```python
from build123d import *

# Parameters (mm, degrees)
F0_W     = 220
F0_H     = 220
F1_DEPTH = 3
F2_W     = 40
F2_H     = 160
F2_R     = 2
F3_DEPTH = 25
F4_SIZE  = 19.99999
F5_R     = 2
F6_DEPTH = 25


# Not quite as in the source:
# - a fillet or chamfer is up to 0.001 mm smaller than in the source, because OpenCascade refuses the exact size
# - a pattern or mirror of a feature is missing from the dataset's text; its kind, count and spacing are read off the source's solid


with BuildPart() as f1:
    # F0 (on Top) → F1 (new body)
    with BuildSketch(Plane.XY):
        Rectangle(F0_W, F0_H)
    extrude(amount=F1_DEPTH)

    # F2 (on face) → F3 (cut)
    with BuildSketch(Plane.XY.offset(3)):
        with Locations((-90, 0)):
            Rectangle(F2_W, F2_H)
        with Locations((105, 105)):
            Circle(F2_R)
        with Locations((105, -105)):
            Circle(F2_R)
        with Locations((-105, 105)):
            Circle(F2_R)
        with Locations((-105, -105)):
            Circle(F2_R)
    f3 = extrude(amount=-F3_DEPTH, mode=Mode.SUBTRACT)

    # F3_copies: F3 across plane
    add(f3.mirror(Plane(origin=(0, 0, 0), x_dir=(0, 0, 1), z_dir=(1, 0, 0))), mode=Mode.SUBTRACT)

    # F4 (size 20 in the source; OpenCascade refuses exactly that, so slightly less here)
    f4_edges = [f1.edges().sort_by_distance(p)[0] for p in [
        (-110, 80, 1.5),
        (-110, -80, 1.5),
        (-70, -80, 1.5),
        (-70, 80, 1.5),
        (110, 80, 1.5),
        (70, 80, 1.5),
        (70, -80, 1.5),
        (110, -80, 1.5),
    ]]
    chamfer(f4_edges, length=F4_SIZE)

    # F5 (on face) → F6 (cut)
    with BuildSketch(Plane(origin=(0, 0, 0), x_dir=(1, 0, 0), z_dir=(0, 0, -1))):
        with Locations((-47, 100)):
            Circle(F5_R)
        with Locations((-47, -40)):
            Circle(F5_R)
        with Locations((47, -40)):
            Circle(F5_R)
        with Locations((47, 100)):
            Circle(F5_R)
    extrude(amount=-F6_DEPTH, mode=Mode.SUBTRACT)


solid = f1.part
```
Build history of the part. All positions in model axes, mm. A direction names the side the tool comes from. Give positions to 0.01 mm unless a question says otherwise; leave off trailing zeros. Loops run counter-clockwise (first coordinate to the right, second up) from the corner with the lowest first, then second, coordinate; pieces in that order, holes last.
Item 1: Slice it at C-C, the plane y = 35. List the corners of the cut face in (x, z).
Answers follow:
outline: (-70, 0) - (70, 0) - (70, 3) - (-70, 3) - close
Item 2: Flat gauge pins, fed straight in: pin 1 (2.5 mm diameter, centred on x = -105, y = 105, fed in from +Z); pin 2 (1.5 mm diameter, centred on y = 20, z = 1.5, fed in from -X); pin 3 (0.9 mm diameter, centred on y = -4.5, z = 1.5, fed in from +X); pin 4 (1.5 mm diameter, centred on y = -62.5, z = 1, fed in from +X). Where does each tip first touch, or does it go through?
Answers follow:
pin 1: passes through
pin 2: stops at x = -70
pin 3: stops at x = 70
pin 4: stops at x = 73.25
Item 3: Slice it at B-B, the plane z = 1.8. Give the number of separate pieces and of enclosed holes in the cut face, and give its area (3 significant figures).
Answers follow:
separate pieces: 1
enclosed holes: 8
area: 35,500 mm2
Item 4: Pull direction Y, two halves, no side cores. Call faces 1 (the face through (100, 90, 2)), 2 (the face through (-2, 2, 0)): released by +Y, released by -Y, zero draft, split by the parting line, or undercut.
Answers follow:
face 1: undercut
face 2: zero draft
Item 5: Slice it at A-A, the plane x = -80.5. List the corners of the cut face in (y, z).
Answers follow:
outline: (-110, 0) - (-70.5, 0) - (-70.5, 3) - (-110, 3) - close; (70.5, 0) - (110, 0) - (110, 3) - (70.5, 3) - close
Item 6: Drill centre lines: line 1 (X direction, y = 40, z = 0.8); line 2 (X direction, y = -105, z = 1.1); line 3 (Y direction, x = 47, z = 1.95). Where is each one in solid material? Low to high.
Answers follow:
line 1: x = -70 to -49, -45 to 45, 49 to 70
line 2: x = -110 to -107, -103 to 103, 107 to 110
line 3: y = -110 to -102, -98 to 38, 42 to 110
Item 7: Which spindle directions (+Z, -Z, +X, -X, +Y, -Y) get a long thin tool onto all of the face, cutting with end or side? Do faces 3 (the face through (-2, 2, 3)), 4 (the face through (80, 70, 2)), 5 (the face through (-100, -90, 2)). Say none if no direction does.
Answers follow:
face 3: +Z, +X, -X, +Y, -Y
face 4: +Z, -Z, +X
face 5: +Z, -Z, -X
